Check sheet for the modelled part. Datum: model origin and axes. Units: mm. A direction names the side the tool comes from. Round coordinates to 2 decimals unless told otherwise and drop trailing zeros. Order: outer loops, then holes, each group sorted by start corner. A loop starts at its lowest first (then second) coordinate and runs counter-clockwise, first axis right, second up.
(1) Mould release check, pull along X, two halves, no side actions. Record for faces 1 (the flat face through (27.214, 0.592, 2.664)), 2 (the flat face through (4.71, 0.592, 13.207)), 3 (the flat face through (0, 2, 8)): released by +X, released by -X, zero draft, split by the parting line, or undercut.
(2) Sectioned sample at A-A, the plane y = 3.15. Count the separate pieces of the cut face and the enclosed holes in it, and give its area (3 significant figures).
(3) Sectioned sample at B-B, the plane x = 27.5. Enter the section's corners in (y, z).
(4) Depth check by flat-ended pin: pin 1 (0.9 mm diameter, centred on x = 12, z = 11, fed in from -Y). Enter the tip coordinate at first touch or a pass-through.
(5) Sectioned sample at D-D, the plane z = 1.5. Enter the section's corners in (x, y).
(6) Thickness scan on probe 1 along X at (y, z) = (0.4, 4.75); probe 2 along Z at (x, y) = (20, 3); probe 3 along Z at (x, y) = (13, 2.65). Record the ranges inside material, lowest first.
(7) Tool access check on faces 4 (the cylindrical face through (19.05, 3.07, 11.27)), 5 (the flat face through (29, 1.2, 13)). Record the directions out of +Z, -Z, +X, -X, +Y, -Y that give a thin tool (end or side, any length) a straight path to the whole face; none if there is none.
```python
from build123d import *

# Parameters (mm, degrees)
SKETCH_W                    = 32
SKETCH_H                    = 16
PAD_DEPTH                   = 5
SKETCH001_R                 = 1.2
HOLE_DEPTH                  = 77.250567
SKETCH001_LINEARPATTERN_2_R = 1.2
HOLE_LINEARPATTERN_2_DEPTH  = 77.250567
SKETCH001_LINEARPATTERN_3_R = 1.2
HOLE_LINEARPATTERN_3_DEPTH  = 77.250567
SKETCH001_LINEARPATTERN_4_R = 1.2
HOLE_LINEARPATTERN_4_DEPTH  = 77.250567
LINEARPATTERN001_COUNT      = 2
LINEARPATTERN001_PITCH      = 8
POCKET_DEPTH                = 1.2
LINEARPATTERN002_COUNT      = 2
LINEARPATTERN002_PITCH      = 8
CHAMFER_SIZE                = 1
CHAMFER001_SIZE             = 2


with BuildPart() as part:
    # Sketch → Pad (new body)
    with BuildSketch(Plane.XZ):
        with Locations((16, 8)):
            Rectangle(SKETCH_W, SKETCH_H)
    extrude(amount=-PAD_DEPTH)

    # Sketch001 (on Face5 of Pad) → Hole (cut, through all)
    with BuildSketch(Plane.XZ):
        with Locations((4, 4)):
            Circle(SKETCH001_R)
    hole = extrude(amount=-HOLE_DEPTH, mode=Mode.SUBTRACT)

    # Sketch001 LinearPattern 2 → Hole LinearPattern 2 (cut, through all)
    with BuildSketch(Plane(origin=(8, 0, 0), x_dir=(1, 0, 0), z_dir=(0, -1, 0))):
        with Locations((4, 4)):
            Circle(SKETCH001_LINEARPATTERN_2_R)
    hole_linearpattern_2 = extrude(amount=-HOLE_LINEARPATTERN_2_DEPTH, mode=Mode.SUBTRACT)

    # Sketch001 LinearPattern 3 → Hole LinearPattern 3 (cut, through all)
    with BuildSketch(Plane(origin=(16, 0, 0), x_dir=(1, 0, 0), z_dir=(0, -1, 0))):
        with Locations((4, 4)):
            Circle(SKETCH001_LINEARPATTERN_3_R)
    hole_linearpattern_3 = extrude(amount=-HOLE_LINEARPATTERN_3_DEPTH, mode=Mode.SUBTRACT)

    # Sketch001 LinearPattern 4 → Hole LinearPattern 4 (cut, through all)
    with BuildSketch(Plane(origin=(24, 0, 0), x_dir=(1, 0, 0), z_dir=(0, -1, 0))):
        with Locations((4, 4)):
            Circle(SKETCH001_LINEARPATTERN_4_R)
    hole_linearpattern_4 = extrude(amount=-HOLE_LINEARPATTERN_4_DEPTH, mode=Mode.SUBTRACT)

    # LinearPattern001: Hole, Hole LinearPattern 2, Hole LinearPattern 3, Hole LinearPattern 4 ×2
    with Locations(*[(0, 0, i * LINEARPATTERN001_PITCH) for i in range(1, LINEARPATTERN001_COUNT)]):
        add(hole, mode=Mode.SUBTRACT)
        add(hole_linearpattern_2, mode=Mode.SUBTRACT)
        add(hole_linearpattern_3, mode=Mode.SUBTRACT)
        add(hole_linearpattern_4, mode=Mode.SUBTRACT)

    # Sketch002 (on Face4 of MultiTransform) → Pocket (cut)
    with BuildSketch(Plane.XZ):
        Polygon((4, 5.616581), (2.6, 4.80829), (2.6, 3.19171), (4, 2.383419), (5.4, 3.19171), (5.4, 4.80829), align=None)
        Polygon((12, 5.674316), (10.55, 4.837158), (10.55, 3.162842), (12, 2.325684), (13.45, 3.162842), (13.45, 4.837158), align=None)
        Polygon((20, 5.732051), (18.5, 4.866025), (18.5, 3.133975), (20, 2.267949), (21.5, 3.133975), (21.5, 4.866025), align=None)
        Polygon((28, 5.789786), (26.45, 4.894893), (26.45, 3.105107), (28, 2.210214), (29.55, 3.105107), (29.55, 4.894893), align=None)
    pocket = extrude(amount=-POCKET_DEPTH, mode=Mode.SUBTRACT)

    # LinearPattern002: Pocket ×2
    with Locations(*[(0, 0, i * LINEARPATTERN002_PITCH) for i in range(1, LINEARPATTERN002_COUNT)]):
        add(pocket, mode=Mode.SUBTRACT)

    # Chamfer
    chamfer_edges = [part.edges().sort_by_distance(p)[0] for p in [
        (0, 2.5, 16),
        (0, 2.5, 0),
    ]]
    chamfer(chamfer_edges, length=CHAMFER_SIZE)

    # Chamfer001
    chamfer001_edges = [part.edges().sort_by_distance(p)[0] for p in [
        (32, 2.5, 16),
        (32, 2.5, 0),
    ]]
    chamfer(chamfer001_edges, length=CHAMFER001_SIZE)


solid = part.part
```
Derived:
1. face 1: undercut
1. face 2: undercut
1. face 3: released by -X
2. separate pieces: 1
2. enclosed holes: 8
2. area: 471 mm2
3. outline: (0, 0) - (5, 0) - (5, 2.91) - (1.2, 2.91) - (1.2, 2.5) - (0, 2.5) - close; (0, 5.5) - (1.2, 5.5) - (1.2, 5.09) - (5, 5.09) - (5, 10.91) - (1.2, 10.91) - (1.2, 10.5) - (0, 10.5) - close; (0, 13.5) - (1.2, 13.5) - (1.2, 13.09) - (5, 13.09) - (5, 16) - (0, 16) - close
4. pin 1: stops at y = 1.2
5. outline: (0, 0) - (31.5, 0) - (31.5, 5) - (0, 5) - close
6. probe 1: x = 0 to 2.6, 5.4 to 10.55, 13.45 to 18.5, 21.5 to 26.45, 29.55 to 32
6. probe 2: z = 0 to 2.8, 5.2 to 10.8, 13.2 to 16
6. probe 3: z = 0 to 3.34, 4.66 to 11.34, 12.66 to 16
7. face 4: +Y, -Y
7. face 5: -Y
